from build123d import *

# Parameters (mm, degrees)
F1_DEPTH = 43.688
F2_R     = 10.859557
F3_DEPTH = 87.377


with BuildPart() as f1:
    # F0 (on Front) → F1 (new body, symmetric)
    with BuildSketch(Plane.XZ):
        Polygon((0, 77.135481), (-18.982824, 20.129664), (-59.417184, 19.798236), (-20.308541, -9.036103), (-48.148591, -42.51045), (0, -15.664687), (61.885897, -42.51045), (29.074408, -9.036103), (71.497343, 19.798236), (24.102971, 19.798236), align=None)
    extrude(amount=F1_DEPTH, both=True)

    # F2 (on face) → F3 (cut, through all)
    with BuildSketch(Plane.XZ.offset(43.688)):
        with Locations((3.072421, 6.236229)):
            Circle(F2_R)
    extrude(amount=-F3_DEPTH, mode=Mode.SUBTRACT)


solid = f1.part
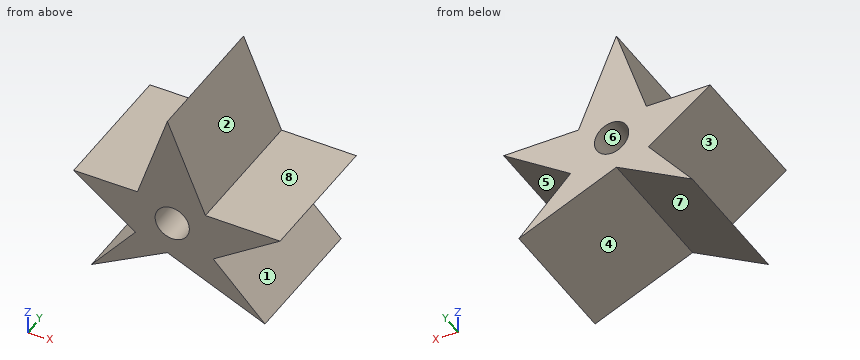
The model under review builds one solid part; all positions refer to its coordinate system, in mm. Face numbers are marked on the shaded views. A direction names the side the tool comes from. Round coordinates to 2 decimals unless told otherwise and drop trailing zeros. Loops run counter-clockwise (first coordinate to the right, second up) from the corner with the lowest first, then second, coordinate; pieces in that order, holes last. Notation, with made-up numbers: (-25.5, 5.5) -> (5.5, 5.5) arc R26 cw to (5.5, 27.5) -> close; hole circle Ø10 at (50, -26.75). An arc over 180 degrees is marked (long way). Write item = value, one per line. Start each with the question number.
Item 1: Take a section at B-B on z = -32.5. Give the boundary of the cut face in (x, y).
Item 2: Take a section at C-C on y = 7. Give the boundary of the cut face in (x, z), plus the area to 3 significant figures.
Item 3: Insertion check: pin 1 (14 mm diameter, centred on x = 43.5, y = 3, fed in from +Z); pin 2 (19.5 mm diameter, centred on x = 3.07, z = 6.24, fed in from +Y); pin 3 (12 mm diameter, centred on x = 52.5, y = 31.5, fed in from -Z); pin 4 (1.5 mm diameter, centred on x = 13.5, y = -20.5, fed in from -Z). Each pin has a flat end and moves straight along its axis. Give the tip position at first contact, or say it passes through.
Item 4: For the marked faces 1, 2, 3 and 4, list the 3-axis set-ups (+Z, -Z, +X, -X, +Y, -Y) from which the entire face can be reached by the end or side of a thin tool; tool diameter is ignored.
Item 5: To check wall thickness, follow L1, parallel to X at y = -17, z = -16; L2, parallel to X at y = 39, z = -22; L3, parallel to Z at x = -42, y = 17.5. State the ranges of each line that lie inside material, in increasing order.
Item 6: Mouldability with a two-part tool opening along X and no side actions: class the marked faces 5, 6, 7 and 8 as released by +X, released by -X, zero draft, split by the parting line, or undercut.
Item 7: Take a section at A-A on x = -35.5. Give the boundary of the cut face in (y, z), plus the area to 3 significant figures.
Item 8: Take a section at D-D on x = 27. Give the boundary of the cut face in (y, z).
Result:
q1.outline = (-39.82, -43.69) -> (-30.19, -43.69) -> (-30.19, 43.69) -> (-39.82, 43.69) -> close; (38.81, -43.69) -> (52.07, -43.69) -> (52.07, 43.69) -> (38.81, 43.69) -> close
q2.outline = (-59.42, 19.8) -> (-20.31, -9.04) -> (-48.15, -42.51) -> (0, -15.66) -> (61.89, -42.51) -> (29.07, -9.04) -> (71.5, 19.8) -> (24.1, 19.8) -> (0, 77.14) -> (-18.98, 20.13) -> close; hole circle Ø21.72 at (3.07, 6.24)
q2.area = 4,670 mm²
q3.pin_1 = 19.8
q3.pin_2 = through
q3.pin_3 = -41.04
q3.pin_4 = -21.85
q4.face_1 = +X, +Y, -Y
q4.face_2 = +Z, +X, +Y, -Y
q4.face_3 = -X, +Y, -Y
q4.face_4 = -Z, +Y, -Y
q5.L1 = -26.1 to -0.6, 0.77 to 35.9
q5.L2 = -31.09 to -11.36, 14.6 to 41.78
q5.L3 = -39.08 to -35.12, 6.96 to 19.94
q6.face_5 = released by +X
q6.face_6 = undercut
q6.face_7 = undercut
q6.face_8 = zero draft
q7.outline = (-43.69, -35.46) -> (43.69, -35.46) -> (43.69, -27.3) -> (-43.69, -27.3) -> close; (-43.69, 2.16) -> (43.69, 2.16) -> (43.69, 19.99) -> (-43.69, 19.99) -> close
q7.area = 2,270 mm²
q8.outline = (-43.69, -27.38) -> (43.69, -27.38) -> (43.69, 19.8) -> (-43.69, 19.8) -> close
